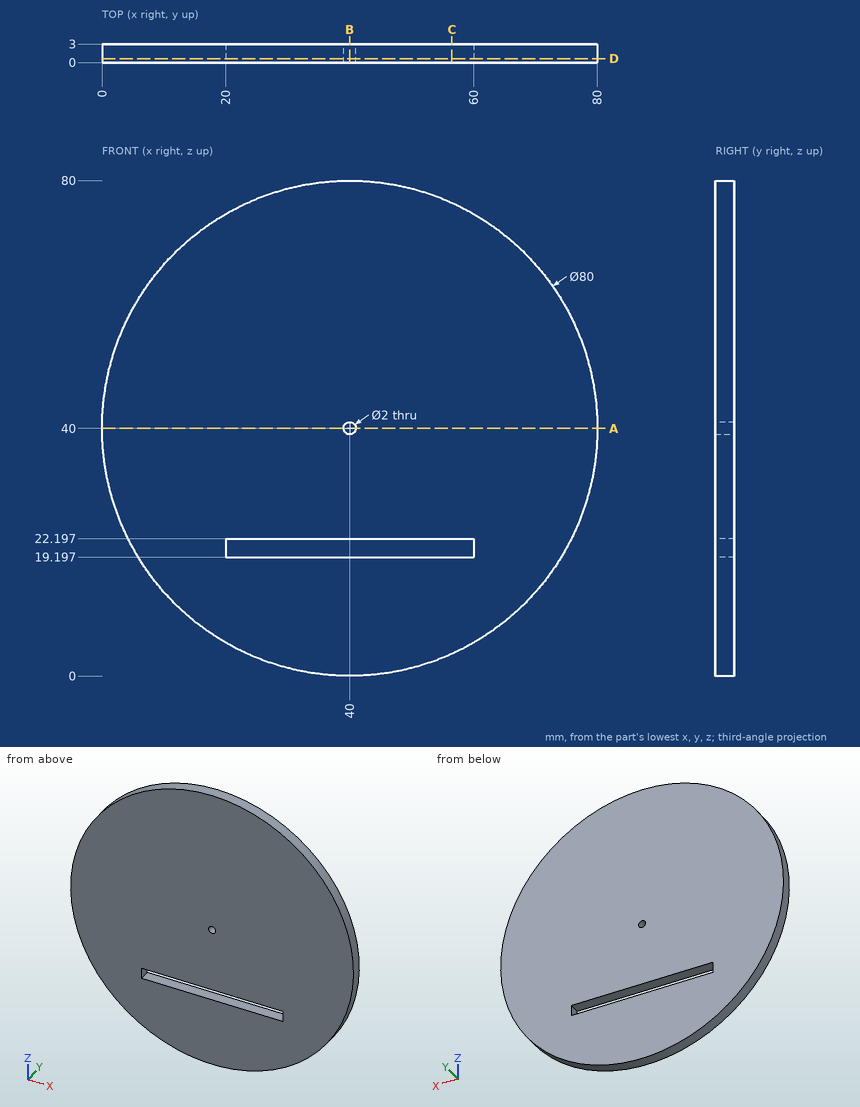
The figure shows three views and two pictorial views of one solid part (mm, origin at its lowest corner). Answer the questions. Give positions to 0.01 mm unless a question says otherwise; leave off trailing zeros. Write each loop counter-clockwise with the first axis right and the second up, starting at its lowest first coordinate (ties: lowest second). Pieces come first, ordered by that corner, then holes.
Q1. The part is cut by section D-D on y = 0.65. Give the vertices of the cut face in (x, z).
Answer:
outline: circle Ø80 at (40, 40); hole (20, 19.2) - (60, 19.2) - (60, 22.2) - (20, 22.2) - close; hole circle Ø2 at (40, 40)
Q2. Given pin 1 (1.5 mm diameter, centred on x = 20.5, y = 1, fed in from -Z); pin 2 (1.5 mm diameter, centred on y = 1.5, z = 20.5, fed in from +X); pin 3 (0.9 mm diameter, centred on x = 49, y = 1.5, fed in from +Z); pin 4 (1.2 mm diameter, centred on x = 40, z = 40, fed in from +Y), each flat-ended and moving along its own axis, determine where each tip first touches the part or whether it passes through.
Answer:
pin 1: stops at z = 4.67
pin 2: stops at x = 75.33
pin 3: stops at z = 79.08
pin 4: passes through
Q3. The part is cut by section A-A on z = 40. Give the vertices of the cut face in (x, y), and give its area (3 significant figures).
Answer:
outline: (0, 0) - (39, 0) - (39, 3) - (0, 3) - close; (41, 0) - (80, 0) - (80, 3) - (41, 3) - close
area: 234 mm2
Q4. Straight lines are drawn through the part: L1, parallel to X at y = 0.65, z = 40; L2, parallel to Z at x = 26.5, y = 1.8; L3, parallel to Z at x = 37.5, y = 1.85. For each, find the intervals that lie inside material, in ascending order.
Answer:
L1: x = 0 to 39, 41 to 80
L2: z = 2.35 to 19.2, 22.2 to 77.65
L3: z = 0.08 to 19.2, 22.2 to 79.92
Q5. The part is cut by section C-C on x = 56.5. Give the vertices of the cut face in (y, z).
Answer:
outline: (0, 3.56) - (3, 3.56) - (3, 19.2) - (0, 19.2) - close; (0, 22.2) - (3, 22.2) - (3, 76.44) - (0, 76.44) - close
Q6. The part is cut by section B-B on x = 40. Give the vertices of the cut face in (y, z).
Answer:
outline: (0, 0) - (3, 0) - (3, 19.2) - (0, 19.2) - close; (0, 22.2) - (3, 22.2) - (3, 39) - (0, 39) - close; (0, 41) - (3, 41) - (3, 80) - (0, 80) - close
